For this review, take the finished solid that the model builds, in its own axes (mm). Face numbers are marked on the shaded views. A direction names the side the tool comes from. Round coordinates to 2 decimals unless told otherwise and drop trailing zeros. Loops run counter-clockwise (first coordinate to the right, second up) from the corner with the lowest first, then second, coordinate; pieces in that order, holes last. Notation, with made-up numbers: (61, 83) -> (92, 83) arc R11 cw to (92, 99) -> close; hole circle Ø10 at (28, 16.25). An arc over 180 degrees is marked (long way). Write each question's results on one line, items separated by ' | '.
Autodesk Inventor part; units mm, degrees
ref_plane "YZ Plane" through (0, 0, 0) normal (1, 0, 0) x (0, 1, 0)
ref_plane "XZ Plane" through (0, 0, 0) normal (0, 1, 0) x (-1, 0, 0)
ref_plane "XY Plane" through (0, 0, 0) normal (0, 0, 1) x (1, 0, 0)
sketch "Sketch1" plane through (0, 0, 0) normal (0, 1, 0) x (-1, 0, 0)
  line L0 (0, 0) -> (-27, 0)
  line L1 (-27, 0) -> (-27, -3)
  line L2 (-27, -3) -> (-22.5, -3)
  line L3 (-22.5, -3) -> (-22.5, -5.5)
  line L4 (-22.5, -5.5) -> (-24.5, -5.5)
  line L5 (-24.5, -5.5) -> (-24.5, -7.5)
  line L6 (-24.5, -7.5) -> (-20.5, -7.5)
  line L7 (-20.5, -7.5) -> (-20.5, -1.5)
  line L8 (-20.5, -1.5) -> (-8, -1.5)
  line L9 (-8, -1.5) -> (-8, -12.5)
  line L10 (-8, -12.5) -> (-6, -12.5)
  line L11 (-6, -12.5) -> (-6, 0)
  line L12 (-6, 0) -> (-6, 3)
  line L13 (-6, 3) -> (-8, 3)
  line L14 (-8, 3) -> (-8, 1.5)
  line L15 (-8, 1.5) -> (-9, 1.5)
  line L16 (-9, 1.5) -> (-10.5, 1.5)
  line L17 (-10.5, 1.5) -> (-10.5, 0)
  line L18 (-27, 0) -> (-27, 1.5)
  line L19 (-27, 1.5) -> (-25.5, 1.5)
  line L20 (-25.5, 1.5) -> (-25.5, 0)
  line L21 (0, -15.6) -> (0, 6.1)
  dimension "d0" = 27
  dimension "d1" = 3
  dimension "d2" = 4.5
  dimension "d3" = 2.5
  dimension "d4" = 2
  dimension "d5" = 2.5
  dimension "d6" = 4
  dimension "d7" = 2
  dimension "d8" = 1.5
  dimension "d9" = 8
  dimension "d10" = 3
  dimension "d11" = 2
  dimension "d12" = 1.5
  dimension "d13" = 1
  dimension "d14" = 1.5
  dimension "d15" = 1.5
  dimension "d16" = 5
revolve "Revolution1" add sketch "Sketch1" angle 360 about axis through (0, 0, -10) along (0, 0, 1)
sketch "Sketch2" plane through (0, 0, 0) normal (0, 0, 1) x (1, 0, 0)
  circle A0 centre (0, 0) radius 10.5
  line L0 (9.5, 1.5) -> (21, 1.5)
  line L1 (22.5, 0) -> (22.5, 0)
  line L2 (21, -1.5) -> (9.5, -1.5)
  line L3 (9.5, -1.5) -> (9.5, 1.5)
  arc A1 (22.5, 0) -> (21, 1.5) centre (21, 0) ccw
  arc A2 (21, -1.5) -> (22.5, 0) centre (21, 0) ccw
  line L4 (7.4772, 6.049) -> (17.4365, 11.799)
  line L5 (19.4856, 11.25) -> (19.4856, 11.25)
  line L6 (18.9365, 9.201) -> (8.9772, 3.451)
  line L7 (8.9772, 3.451) -> (7.4772, 6.049)
  arc A3 (19.4856, 11.25) -> (17.4365, 11.799) centre (18.1865, 10.5) ccw
  arc A4 (18.9365, 9.201) -> (19.4856, 11.25) centre (18.1865, 10.5) ccw
  line L8 (3.451, 8.9772) -> (9.201, 18.9365)
  line L9 (11.25, 19.4856) -> (11.25, 19.4856)
  line L10 (11.799, 17.4365) -> (6.049, 7.4772)
  line L11 (6.049, 7.4772) -> (3.451, 8.9772)
  arc A5 (11.25, 19.4856) -> (9.201, 18.9365) centre (10.5, 18.1865) ccw
  arc A6 (11.799, 17.4365) -> (11.25, 19.4856) centre (10.5, 18.1865) ccw
  line L12 (-1.5, 9.5) -> (-1.5, 21)
  line L13 (0, 22.5) -> (0, 22.5)
  line L14 (1.5, 21) -> (1.5, 9.5)
  line L15 (1.5, 9.5) -> (-1.5, 9.5)
  arc A7 (0, 22.5) -> (-1.5, 21) centre (0, 21) ccw
  arc A8 (1.5, 21) -> (0, 22.5) centre (0, 21) ccw
  line L16 (-6.049, 7.4772) -> (-11.799, 17.4365)
  line L17 (-11.25, 19.4856) -> (-11.25, 19.4856)
  line L18 (-9.201, 18.9365) -> (-3.451, 8.9772)
  line L19 (-3.451, 8.9772) -> (-6.049, 7.4772)
  arc A9 (-11.25, 19.4856) -> (-11.799, 17.4365) centre (-10.5, 18.1865) ccw
  arc A10 (-9.201, 18.9365) -> (-11.25, 19.4856) centre (-10.5, 18.1865) ccw
  line L20 (-8.9772, 3.451) -> (-18.9365, 9.201)
  line L21 (-19.4856, 11.25) -> (-19.4856, 11.25)
  line L22 (-17.4365, 11.799) -> (-7.4772, 6.049)
  line L23 (-7.4772, 6.049) -> (-8.9772, 3.451)
  arc A11 (-19.4856, 11.25) -> (-18.9365, 9.201) centre (-18.1865, 10.5) ccw
  arc A12 (-17.4365, 11.799) -> (-19.4856, 11.25) centre (-18.1865, 10.5) ccw
  line L24 (-9.5, -1.5) -> (-21, -1.5)
  line L25 (-22.5, 0) -> (-22.5, 0)
  line L26 (-21, 1.5) -> (-9.5, 1.5)
  line L27 (-9.5, 1.5) -> (-9.5, -1.5)
  arc A13 (-22.5, 0) -> (-21, -1.5) centre (-21, 0) ccw
  arc A14 (-21, 1.5) -> (-22.5, 0) centre (-21, 0) ccw
  line L28 (-7.4772, -6.049) -> (-17.4365, -11.799)
  line L29 (-19.4856, -11.25) -> (-19.4856, -11.25)
  line L30 (-18.9365, -9.201) -> (-8.9772, -3.451)
  line L31 (-8.9772, -3.451) -> (-7.4772, -6.049)
  arc A15 (-19.4856, -11.25) -> (-17.4365, -11.799) centre (-18.1865, -10.5) ccw
  arc A16 (-18.9365, -9.201) -> (-19.4856, -11.25) centre (-18.1865, -10.5) ccw
  line L32 (-3.451, -8.9772) -> (-9.201, -18.9365)
  line L33 (-11.25, -19.4856) -> (-11.25, -19.4856)
  line L34 (-11.799, -17.4365) -> (-6.049, -7.4772)
  line L35 (-6.049, -7.4772) -> (-3.451, -8.9772)
  arc A17 (-11.25, -19.4856) -> (-9.201, -18.9365) centre (-10.5, -18.1865) ccw
  arc A18 (-11.799, -17.4365) -> (-11.25, -19.4856) centre (-10.5, -18.1865) ccw
  line L36 (1.5, -9.5) -> (1.5, -21)
  line L37 (0, -22.5) -> (0, -22.5)
  line L38 (-1.5, -21) -> (-1.5, -9.5)
  line L39 (-1.5, -9.5) -> (1.5, -9.5)
  arc A19 (0, -22.5) -> (1.5, -21) centre (0, -21) ccw
  arc A20 (-1.5, -21) -> (0, -22.5) centre (0, -21) ccw
  line L40 (6.049, -7.4772) -> (11.799, -17.4365)
  line L41 (11.25, -19.4856) -> (11.25, -19.4856)
  line L42 (9.201, -18.9365) -> (3.451, -8.9772)
  line L43 (3.451, -8.9772) -> (6.049, -7.4772)
  arc A21 (11.25, -19.4856) -> (11.799, -17.4365) centre (10.5, -18.1865) ccw
  arc A22 (9.201, -18.9365) -> (11.25, -19.4856) centre (10.5, -18.1865) ccw
  line L44 (8.9772, -3.451) -> (18.9365, -9.201)
  line L45 (19.4856, -11.25) -> (19.4856, -11.25)
  line L46 (17.4365, -11.799) -> (7.4772, -6.049)
  line L47 (7.4772, -6.049) -> (8.9772, -3.451)
  arc A23 (19.4856, -11.25) -> (18.9365, -9.201) centre (18.1865, -10.5) ccw
  arc A24 (17.4365, -11.799) -> (19.4856, -11.25) centre (18.1865, -10.5) ccw
  point P0 (22.5, -1.5)
  point P1 (20.2356, 9.951)
  point P2 (12.549, 18.7356)
  point P3 (1.5, 22.5)
  point P4 (-9.951, 20.2356)
  point P5 (-18.7356, 12.549)
  point P6 (-22.5, 1.5)
  point P7 (-20.2356, -9.951)
  point P8 (-12.549, -18.7356)
  point P9 (-1.5, -22.5)
  point P10 (9.951, -20.2356)
  point P11 (18.7356, -12.549)
  dimension "d18" = 13
  dimension "d19" = 1
  dimension "d20" = 3
  dimension "d21" = 1.5
  dimension "d22" = 1.5
  dimension "d25" = 360
extrude "Extrusion1" add sketch "Sketch2" along normal blind 1 contours A0 L2 L3 L0 | A0 L0 A1 A2 L2 | L6 L7 L4 A0 | A0 L4 A3 A4 L6 | L44 A23 A24 L46 A0 | A0 L46 L47 L44 | L10 L11 L8 A0 | A0 L8 A5 A6 L10 | L40 A21 A22 L42 A0 | A0 L42 L43 L40 | L14 L15 L12 A0 | A0 L12 A7 A8 L14 | L36 A19 A20 L38 A0 | A0 L38 L39 L36 | L18 L19 L16 A0 | A0 L16 A9 A10 L18 | L32 A17 A18 L34 A0 | A0 L34 L35 L32 | L22 L23 L20 A0 | A0 L20 A11 A12 L22 | L28 A15 A16 L30 A0 | A0 L30 L31 L28 | L26 L27 L24 A0 | A0 L24 A13 A14 L26
sketch "Sketch3" plane through (0, 0, 0) normal (0, 1, 0) x (-1, 0, 0)
  line L0 (24.5, -5.5) -> (-24.5, -5.5)
  line L1 (22.4583, -5.5) -> (24.4583, -5.5)
  line L2 (24.4583, -5.5) -> (24.4583, -3)
  line L3 (24.4583, -3) -> (22.4583, -3)
  line L4 (22.4583, -3) -> (22.4583, -5.5)
  point P0 (0, 0)
  dimension "d29" = 2
  dimension "d30" = 2.5
extrude "Extrusion2" add sketch "Sketch3" against normal blind 1
properties part number "MotorGrill"
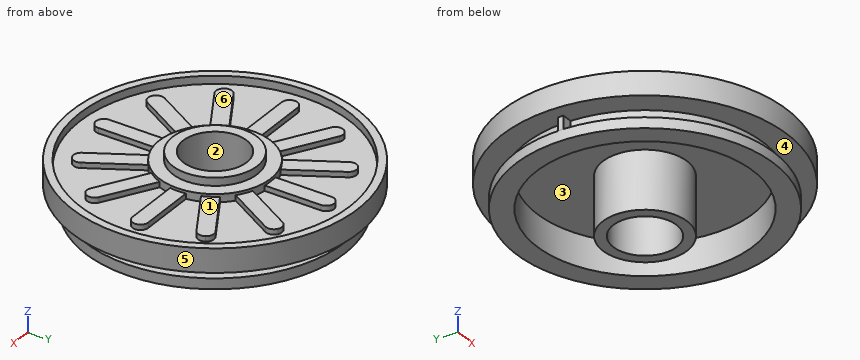
1. Consider section C-C (z = -8.75). State the section outline as (x, y) points, plus the area to 3 significant figures.
Values found:
outline: circle Ø16 at (0, 0); hole circle Ø12 at (0, 0) | area: 88.0 mm2
2. To check wall thickness, follow probe 1 along Y at (x, z) = (0, -2.75); probe 2 along Y at (x, z) = (0, 0.7); probe 3 along Z at (x, y) = (-17.5, 19.5). State the ranges of each line that lie inside material, in increasing order.
Values found:
probe 1: y = -27 to -20.5, -8 to -6, 6 to 8, 20.5 to 27 | probe 2: y = -27 to -25.5, -22.5 to -6, 6 to 22.5, 25.5 to 27 | probe 3: z = -3 to 1.5
3. Consider section A-A (z = -4). State the section outline as (x, y) points, plus the area to 3 significant figures.
Values found:
outline: (-24.46, -1) -> (-22.48, -1) arc R22.5 ccw (long way) to (-22.5, 0) -> (-24.46, 0) -> close; circle Ø16 at (0, 0); hole circle Ø41 at (0, 0); hole circle Ø12 at (0, 0) | area: 360 mm2
4. For pin 1 (6 mm diameter, centred on y = 21, z = -0.5, fed in from -X); pin 2 (1 mm diameter, centred on x = 5.5, y = 14, fed in from +Z); pin 3 (2.5 mm diameter, centred on x = 0, y = 15.5, fed in from +Z), all flat-tipped, find the tip position at first contact; note any pin that passes through.
Values found:
pin 1: stops at x = -20.12 | pin 2: stops at z = 0 | pin 3: stops at z = 1
5. Consider section B-B (z = -0.75). State the section outline as (x, y) points.
Values found:
outline: circle Ø54 at (0, 0); hole circle Ø12 at (0, 0)
6. Tool access review of the marked faces 1, 2 and 3: name each direction out of +Z, -Z, +X, -X, +Y, -Y from which nothing blocks a thin tool from reaching the whole face with its end or side.
Values found:
face 1: +Z | face 2: +Z, -Z | face 3: -Z
7. Draft analysis for pull direction X (two halves, no side actions). For the marked faces 4, 5 and 6, state which applies: released by +X, released by -X, zero draft, split by the parting line, or undercut.
Values found:
face 4: zero draft | face 5: split by the parting line | face 6: undercut
